Geometry check sheet. Reference: the model listing, model coordinates, mm. A direction names the side the tool comes from. Coordinates: 2 decimals unless noted, no trailing zeros. Write each loop counter-clockwise with the first axis right and the second up, starting at its lowest first coordinate (ties: lowest second). Pieces come first, ordered by that corner, then holes. Notation, with made-up numbers: (-25.75, -24.75) -> (-17.75, -24.75) arc R19 cw to (-17.75, 7.25) -> close; hole circle Ø5 at (14, 75). An arc over 180 degrees is marked (long way). Answer in a Markdown table with one row per item. Add a question column.
Q1. Section check C-C, the plane z = -7.75. Record the boundary of the cut face in (x, y), and give its area (3 significant figures).
Q2. Section check B-B, the plane y = 1.85. Record the boundary of the cut face in (x, z), and give its area (3 significant figures).
Q3. Release check for a two-part mould opening along X. For faces 1 (the face through (4.383, 1, -6)), 2 (the face through (0.883, 2.5, -6.3)), 3 (the face through (1.8, 0.5, -1.852)), 4 (the face through (-0.617, 1, -6)) record: pulls with the +X half, pulls with the -X half, needs draft (parallel to the pull), parting line crosses it, or undercut.
Q4. Tool access check on faces 5 (the face through (2.883, 2.5, -6.3)), 6 (the face through (1.8, 0.8, -8.852)), 7 (the face through (3.683, 1.5, -6.4)), 8 (the face through (2, 0, -5)), 9 (the face through (0, 2.2, -3.852)). Record the directions out of +Z, -Z, +X, -X, +Y, -Y that give a thin tool (end or side, any length) a straight path to the whole face; none if there is none.
Q5. Thickness scan on line 1 (X direction, y = 2.05, z = -4.5); line 2 (X direction, y = 1.3, z = -8.25); line 3 (Y direction, x = 1.85, z = -8.5). Record the ranges inside material, lowest first.
Q6. Section check A-A, the plane x = 3.1. Record the boundary of the cut face in (y, z).
Q7. Gauge pin test, flat ends, axial feed: P1, Ø1.6, axis at x = 0.5, y = 2.5, coming from the +Z side; P2, Ø0.9, axis at x = 3.5, z = -7.5, coming from the -Y side. Record the tip position at first contact, or that the pin passes through.
Q8. Section check D-D, the plane z = -3.75. Record the boundary of the cut face in (x, y).
```python
from build123d import *

# Parameters (mm, degrees)
SKETCH1_W           = 5
SKETCH1_H           = 7
BOSS_EXTRUDE1_DEPTH = 3
SKETCH2_W           = 2
SKETCH2_H           = 7
CUT_EXTRUDE1_DEPTH  = 2
SKETCH3_W           = 3.6
SKETCH3_H           = 1
CUT_EXTRUDE2_DEPTH  = 9.786829282
SKETCH4_W           = 5
SKETCH4_H           = 2
CUT_EXTRUDE3_DEPTH  = 2


with BuildPart() as part:
    # Sketch1 → Boss-Extrude1 (new body)
    with BuildSketch(Plane(origin=(0, 0, 0), x_dir=(1, 0, 0), z_dir=(0, 1, 0))):
        with Locations((1.882735313, 5.351794061)):
            Rectangle(SKETCH1_W, SKETCH1_H)
    extrude(amount=BOSS_EXTRUDE1_DEPTH)

    # Sketch2 → Cut-Extrude1 (cut)
    with BuildSketch(Plane(origin=(0, 3, 0), x_dir=(1, 0, 0), z_dir=(0, 1, 0))):
        with Locations((1.882735313, 5.351794061)):
            Rectangle(SKETCH2_W, SKETCH2_H)
    extrude(amount=-CUT_EXTRUDE1_DEPTH, mode=Mode.SUBTRACT)

    # Sketch3 → Cut-Extrude2 (cut, through all)
    with BuildSketch(Plane(origin=(0, 0, -8.851794061), x_dir=(-1, 0, 0), z_dir=(0, 0, -1))):
        with Locations((-1.882735313, 1.5)):
            Rectangle(SKETCH3_W, SKETCH3_H)
    extrude(amount=-CUT_EXTRUDE2_DEPTH, mode=Mode.SUBTRACT)

    # Sketch4 → Cut-Extrude3 (cut)
    with BuildSketch(Plane.XY.offset(-1.851794061)):
        with Locations((1.882735313, 2)):
            Rectangle(SKETCH4_W, SKETCH4_H)
    extrude(amount=-CUT_EXTRUDE3_DEPTH, mode=Mode.SUBTRACT)


solid = part.part
```
Calculated:
| question | item | result |
|---|---|---|
| 1 | outline | (-0.62, 0) -> (4.38, 0) -> (4.38, 3) -> (2.88, 3) -> (2.88, 2) -> (3.68, 2) -> (3.68, 1) -> (0.08, 1) -> (0.08, 2) -> (0.88, 2) -> (0.88, 3) -> (-0.62, 3) -> close |
| 1 | area | 9.40 mm² |
| 2 | outline | (-0.62, -8.85) -> (0.08, -8.85) -> (0.08, -3.85) -> (-0.62, -3.85) -> close; (3.68, -8.85) -> (4.38, -8.85) -> (4.38, -3.85) -> (3.68, -3.85) -> close |
| 2 | area | 7.00 mm² |
| 3 | face 1 | pulls with the +X half |
| 3 | face 2 | undercut |
| 3 | face 3 | needs draft |
| 3 | face 4 | pulls with the -X half |
| 4 | face 5 | +Z, -Z, +Y |
| 4 | face 6 | -Z, +X, -X, +Y, -Y |
| 4 | face 7 | +Z, -Z |
| 4 | face 8 | +Z, -Z, +X, -X, -Y |
| 4 | face 9 | +Z, +X, -X, +Y |
| 5 | line 1 | x = -0.62 to 0.88, 2.88 to 4.38 |
| 5 | line 2 | x = -0.62 to 0.08, 3.68 to 4.38 |
| 5 | line 3 | y = 0 to 1 |
| 6 | outline | (0, -8.85) -> (1, -8.85) -> (1, -1.85) -> (0, -1.85) -> close; (2, -8.85) -> (3, -8.85) -> (3, -3.85) -> (2, -3.85) -> close |
| 7 | P1 | stops at z = -3.85 |
| 7 | P2 | stops at y = 0 |
| 8 | outline | (-0.62, 0) -> (4.38, 0) -> (4.38, 1) -> (-0.62, 1) -> close |
